```python
from build123d import *

# Parameters (mm, degrees)
SKETCH1_W                   = 203.2
SKETCH1_H                   = 101.6
BOSS_EXTRUDE1_DEPTH         = 6.35
F_1_4_0_25_DIAMETER_HOLE1_D = 6.35
FILLET1_R                   = 6.35


with BuildPart() as part:
    # Sketch1 → Boss-Extrude1 (new body)
    with BuildSketch(Plane(origin=(0, 0, 0), x_dir=(1, 0, 0), z_dir=(0, 1, 0))):
        with Locations((101.6, 50.8)):
            Rectangle(SKETCH1_W, SKETCH1_H)
    extrude(amount=BOSS_EXTRUDE1_DEPTH)

    # 1/4 (0.25) Diameter Hole1 (through all)
    with Locations(Plane(origin=(0, 6.35, 0), x_dir=(1, 0, 0), z_dir=(0, 1, 0))):
        with Locations((61.726765383, 55.793470503), (131.576765383, 55.793470503)):
            Hole(F_1_4_0_25_DIAMETER_HOLE1_D / 2)

    # Fillet1
    fillet1_edges = [part.edges().sort_by_distance(p)[0] for p in [
        (0, 3.175, -101.6),
        (203.2, 3.175, -101.6),
        (203.2, 3.175, 0),
        (0, 3.175, 0),
    ]]
    fillet(fillet1_edges, radius=FILLET1_R)


solid = part.part
```
Input: part model. Units: mm. Frame: model coordinates. Give positions to 0.01 mm unless a question says otherwise; leave off trailing zeros. Order: outer loops, then holes, each group sorted by start corner. A loop starts at its lowest first (then second) coordinate and runs counter-clockwise, first axis right, second up. Notation, with made-up numbers: (56.5, 78) - (77.5, 78) arc R25 cw to (77.5, 93) - close; hole circle Ø3 at (46.5, 59). An arc over 180 degrees is marked (long way). One line per item, written item: value.
1. Draft query along X for faces 1 (the face through (201.29, 3.22, -1.81)), 2 (the face through (64.1, 3.1, -57.9)), 3 (the face through (131.99, 3.13, -58.94)), 4 (the face through (0, 3, -50)). Return one class per face: released by +X, released by -X, zero draft, split by the parting line, or undercut.
Determined:
face 1: released by +X
face 2: undercut
face 3: undercut
face 4: released by -X
2. Cut plane A-A, the plane x = 130.5. Output: boundary loops of the cut face in (y, z), and give its area (3 significant figures).
Determined:
outline: (0, -101.6) - (6.35, -101.6) - (6.35, -58.78) - (0, -58.78) - close; (0, -52.81) - (6.35, -52.81) - (6.35, 0) - (0, 0) - close
area: 607 mm2
3. Line query: probe 1 along X at (y, z) = (4.25, -4.5). Output: solid intervals per line, ascending.
Determined:
probe 1: 0.28 to 202.92
